Verification items for the finished model (mm, model axes). A direction names the side the tool comes from. Give positions to 0.01 mm unless a question says otherwise; leave off trailing zeros. Loops run counter-clockwise (first coordinate to the right, second up) from the corner with the lowest first, then second, coordinate; pieces in that order, holes last. Notation, with made-up numbers: (44.5, 84) - (72.5, 84) arc R25 ccw to (72.5, 103) - close; hole circle Ø8 at (25.25, 40). An arc over 180 degrees is marked (long way). Put each result on its own line as item: value. Start each with the question number.
```python
from build123d import *

# Parameters (mm, degrees)
BOX004_W        = 21
BOX004_H        = 4
BOX004_DEPTH    = 10
BOX003_W        = 15
BOX003_H        = 4
BOX003_DEPTH    = 19
BOX_W           = 15
BOX_H           = 4
BOX_DEPTH       = 19
BOX002_W        = 15
BOX002_H        = 8
BOX002_DEPTH    = 10
BOX001_W        = 27
BOX001_H        = 8
BOX001_DEPTH    = 16
FILLET_R        = 2
FILLET001_R     = 2
CHAMFER_SIZE    = 1
CHAMFER001_SIZE = 1
CHAMFER002_SIZE = 0.4


with BuildPart() as cube004:
    # Box004 → Box004 (new body)
    with BuildSketch(Plane(origin=(-3, 2, 13), x_dir=(1, 0, 0), z_dir=(0, 0, 1))):
        with Locations((10.5, 2)):
            Rectangle(BOX004_W, BOX004_H)
    extrude(amount=BOX004_DEPTH)


with BuildPart() as cube003:
    # Box003 → Box003 (new body)
    with BuildSketch(Plane(origin=(18, 2, 0), x_dir=(1, 0, 0), z_dir=(0, 0, 1))):
        with Locations((7.5, 2)):
            Rectangle(BOX003_W, BOX003_H)
    extrude(amount=BOX003_DEPTH)


with BuildPart() as fusion:
    # Box → Box (new body)
    with BuildSketch(Plane(origin=(-18, 2, 0), x_dir=(1, 0, 0), z_dir=(0, 0, 1))):
        with Locations((7.5, 2)):
            Rectangle(BOX_W, BOX_H)
    extrude(amount=BOX_DEPTH)

    # Fusion: union Cube004, Cube003
    add(cube004.part)
    add(cube003.part)


with BuildPart() as cube002:
    # Box002 → Box002 (new body)
    with BuildSketch(Plane.XY):
        with Locations((7.5, 4)):
            Rectangle(BOX002_W, BOX002_H)
    extrude(amount=BOX002_DEPTH)


with BuildPart() as f_10x15_hole:
    # Box001 → Box001 (new body)
    with BuildSketch(Plane(origin=(-6, 0, 0), x_dir=(1, 0, 0), z_dir=(0, 0, 1))):
        with Locations((13.5, 4)):
            Rectangle(BOX001_W, BOX001_H)
    extrude(amount=BOX001_DEPTH)

    # Cut: cut Cube002
    add(cube002.part, mode=Mode.SUBTRACT)

    # Cut001: cut Fusion
    add(fusion.part, mode=Mode.SUBTRACT)

    # Fillet
    fillet_edges = [f_10x15_hole.edges().sort_by_distance(p)[0] for p in [
        (0, 4, 10),
        (15, 4, 10),
    ]]
    fillet(fillet_edges, radius=FILLET_R)

    # Fillet001
    fillet001_edges = [f_10x15_hole.edges().sort_by_distance(p)[0] for p in [
        (-6, 1, 16),
        (21, 1, 16),
        (-6, 7, 16),
        (21, 7, 16),
    ]]
    fillet(fillet001_edges, radius=FILLET001_R)

    # Chamfer
    chamfer_edges = [f_10x15_hole.edges().sort_by_distance(p)[0] for p in [
        (-3, 4, 13),
        (18, 4, 13),
    ]]
    chamfer(chamfer_edges, length=CHAMFER_SIZE)

    # Chamfer001
    chamfer001_edges = [f_10x15_hole.edges().sort_by_distance(p)[0] for p in [
        (15, 8, 4),
        (14.414214, 8, 9.414214),
        (7.5, 8, 10),
        (0.585786, 8, 9.414214),
        (0, 8, 4),
        (0, 0, 4),
        (15, 0, 4),
        (14.414214, 0, 9.414214),
        (7.5, 0, 10),
        (0.585786, 0, 9.414214),
    ]]
    chamfer(chamfer001_edges, length=CHAMFER001_SIZE)

    # Chamfer002
    chamfer002_edges = [f_10x15_hole.edges().sort_by_distance(p)[0] for p in [
        (-6, 8, 7),
        (-5.414214, 8, 15.414214),
        (7.5, 8, 16),
        (20.414214, 8, 15.414214),
        (21, 8, 7),
        (-6, 0, 7),
        (-5.414214, 0, 15.414214),
        (7.5, 0, 16),
        (20.414214, 0, 15.414214),
        (21, 0, 7),
    ]]
    chamfer(chamfer002_edges, length=CHAMFER002_SIZE)


solid = f_10x15_hole.part
```
1) Section check B-B, the plane y = 6.5. Enter the section's corners in (x, z), plus the area to 3 significant figures.
2) Section check D-D, the plane z = 13.5. Enter the section's corners in (x, y).
3) Set-up check for faces 4 (the face through (-2.5, 4, 12.5)), 5 (the face through (0, 4, 4)), 6 (the face through (-0.5, 7.5, 4.1)), 7 (the face through (14.666, 0.618, 9.703)): record each of +Z, -Z, +X, -X, +Y, -Y from which the full face is reachable in a straight line by a thin tool's end or side.
4) Depth check by flat-ended pin: P1, Ø1.2, axis at x = 5, y = 4.5, coming from the +Z side; P2, Ø1.2, axis at y = 4, z = 7, coming from the -X side; P3, Ø2, axis at y = 4.5, z = 9, coming from the +X side; P4, Ø5, axis at x = 3.5, z = 6, coming from the -Y side. Enter the tip coordinate at first touch or a pass-through.
5) Section check A-A, the plane z = 7.25. Enter the section's corners in (x, y), plus the area to 3 significant figures.
6) Scan lines: line 1 along X through (y, z) = (1.5, 1.5); line 2 along Y through (x, z) = (18.5, 14.5); line 3 along Z through (x, y) = (12, 5.25). Record each from-to range of solid material in increasing order. Write a range as from..to.
7) Draft check along X on faces 1 (the face through (-5.43, 1.21, 15.4)), 2 (the face through (14.4, 4.04, 9.43)), 3 (the face through (7.3, 2, 13.2)). Enter one of: pulls with the +X half, pulls with the -X half, needs draft (parallel to the pull), parting line crosses it, or undercut.
8) Section check C-C, the plane x = 11.5. Enter the section's corners in (y, z).
Results are:
1. outline: (-6, 0) - (0, 0) - (0, 8) arc R2 cw to (2, 10) - (13, 10) arc R2 cw to (15, 8) - (15, 0) - (21, 0) - (21, 14) arc R2 ccw to (19, 16) - (-4, 16) arc R2 ccw to (-6, 14) - close
1. area: 282 mm2
2. outline: (-6, 0.4) - (-5.6, 0) - (20.6, 0) - (21, 0.4) - (21, 2) - (-6, 2) - close; (-6, 6) - (21, 6) - (21, 7.6) - (20.6, 8) - (-5.6, 8) - (-6, 7.6) - close
3. face 4: +Z, -X
3. face 5: -Z, +Y, -Y
3. face 6: -Z, +Y
3. face 7: -Z, -Y
4. P1: stops at z = 13
4. P2: stops at x = -3
4. P3: stops at x = 18
4. P4: passes through
5. outline: (-6, 0.4) - (-5.6, 0) - (-1, 0) - (0, 1) - (0, 7) - (-1, 8) - (-5.6, 8) - (-6, 7.6) - (-6, 6) - (-3, 6) - (-3, 2) - (-6, 2) - close; (15, 1) - (16, 0) - (20.6, 0) - (21, 0.4) - (21, 2) - (18, 2) - (18, 6) - (21, 6) - (21, 7.6) - (20.6, 8) - (16, 8) - (15, 7) - close
5. area: 69.7 mm2
6. line 1: x = -6..0, 15..21
6. line 2: y = 0..2, 6..8
6. line 3: z = 10..13
7. face 1: pulls with the -X half
7. face 2: undercut
7. face 3: needs draft
8. outline: (0, 11) - (1, 10) - (7, 10) - (8, 11) - (8, 15.6) - (7.6, 16) - (6, 16) - (6, 13) - (2, 13) - (2, 16) - (0.4, 16) - (0, 15.6) - close
